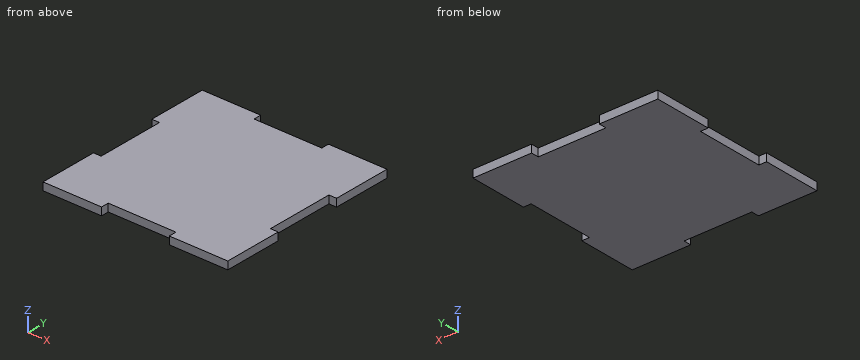
Autodesk Inventor part; units mm, degrees
ref_plane "YZ Plane" through (0, 0, 0) normal (1, 0, 0) x (0, 1, 0)
ref_plane "XZ Plane" through (0, 0, 0) normal (0, 1, 0) x (-1, 0, 0)
ref_plane "XY Plane" through (0, 0, 0) normal (0, 0, 1) x (1, 0, 0)
sketch "Sketch1" plane through (0, 0, 0) normal (0, 0, 1) x (1, 0, 0)
  line L0 (12.7, -31.75) -> (12.7, -34.6456)
  line L1 (12.7, -34.6456) -> (34.6456, -34.6456)
  line L2 (34.6456, -34.6456) -> (34.6456, -12.7)
  line L3 (34.6456, -12.7) -> (31.75, -12.7)
  line L4 (31.75, -12.7) -> (31.75, 12.7)
  line L5 (31.75, 12.7) -> (34.6456, 12.7)
  line L6 (34.6456, 12.7) -> (34.6456, 34.6456)
  line L7 (34.6456, 34.6456) -> (12.7, 34.6456)
  line L8 (12.7, 34.6456) -> (12.7, 31.75)
  line L9 (12.7, 31.75) -> (-12.7, 31.75)
  line L10 (-12.7, 31.75) -> (-12.7, 34.6456)
  line L11 (-12.7, 34.6456) -> (-34.6456, 34.6456)
  line L12 (-34.6456, 34.6456) -> (-34.6456, 12.7)
  line L13 (-34.6456, 12.7) -> (-31.75, 12.7)
  line L14 (-31.75, 12.7) -> (-31.75, -12.7)
  line L15 (-31.75, -12.7) -> (-34.6456, -12.7)
  line L16 (-34.6456, -12.7) -> (-34.6456, -34.6456)
  line L17 (-34.6456, -34.6456) -> (-12.7, -34.6456)
  line L18 (-12.7, -34.6456) -> (-12.7, -31.75)
  line L19 (-12.7, -31.75) -> (12.7, -31.75)
  point P0 (0, 0)
extrude "Extrusion1" add sketch "Sketch1" along normal blind 2.8956
properties part number "outside_box_top_bot" material "Polycarbonate, Clear"
Here's how the part is built. I have some questions about the finished solid (model axes, mm). Round coordinates to 2 decimals unless told otherwise and drop trailing zeros. Loops run counter-clockwise (first coordinate to the right, second up) from the corner with the lowest first, then second, coordinate; pieces in that order, holes last. Notation, with made-up numbers: M -30.5,-25.75 L -25.5,-25.75 A23 cw -25.5,-3.75 Z; hole C 58,87 d9. An arc over 180 degrees is marked long. Write each question's results on one line, items separated by ' | '. Start each with the question number.
(1) Will this pin go through, and if not, where does the flat tip stop? P1, Ø1.4, axis at y = 3, z = 1.5, coming from the -X side.
(2) If I drill on probe 1 along X at (y, z) = (-10, 2.3), over which ranges is the centre line in solid material (lowest first)? Write a range as from..to.
(3) I want a section at B-B (x = -4). Please give me the cut outline in (y, z), then the cut area to 3 significant figures.
(4) I want a section at A-A (z = 2.4). Please give me the cut outline in (x, y), then the cut area to 3 significant figures.
Solved:
1) P1: stops at x = -31.75
2) probe 1: x = -31.75..31.75
3) outline: M -31.75,0 L 31.75,0 L 31.75,2.9 L -31.75,2.9 Z | area: 184 mm²
4) outline: M -34.65,-34.65 L -12.7,-34.65 L -12.7,-31.75 L 12.7,-31.75 L 12.7,-34.65 L 34.65,-34.65 L 34.65,-12.7 L 31.75,-12.7 L 31.75,12.7 L 34.65,12.7 L 34.65,34.65 L 12.7,34.65 L 12.7,31.75 L -12.7,31.75 L -12.7,34.65 L -34.65,34.65 L -34.65,12.7 L -31.75,12.7 L -31.75,-12.7 L -34.65,-12.7 Z | area: 4,510 mm²
